```python
from build123d import *

# Parameters (mm, degrees)
SKETCH2_W               = 6.35
SKETCH2_H               = 50.8
SKETCH2_W_2             = 2.54
SKETCH2_W_3             = 31.75
SKETCH2_W_4             = 3.81
SKETCH2_W_5             = 12.7
BOSS_EXTRUDE2_DEPTH     = 73.66
CUT_EXTRUDE2_DEPTH      = 26.4
CUT_EXTRUDE2_DEPTH_BACK = 77.2
CUT_EXTRUDE3_DEPTH      = 22.86
CUT_EXTRUDE4_DEPTH      = 38.1


with BuildPart() as part:
    # Sketch2 → Boss-Extrude2 (new body)
    with BuildSketch(Plane.XY):
        with Locations((98.925952955, 12.684680338)):
            Rectangle(SKETCH2_W, SKETCH2_H)
        with Locations((105.275952955, 12.684680338)):
            Rectangle(SKETCH2_W, SKETCH2_H)
        with Locations((109.720952955, 12.684680338)):
            Rectangle(SKETCH2_W_2, SKETCH2_H)
        with Locations((79.875952955, 12.684680338)):
            Rectangle(SKETCH2_W_3, SKETCH2_H)
        with Locations((62.095952955, 12.684680338)):
            Rectangle(SKETCH2_W_4, SKETCH2_H)
        Polygon((-28.709047045, -38.115319662), (60.190952955, -38.115319662), (60.190952955, 63.484680338), (-28.709047045, 63.484680338), (-28.709047045, -12.715319662), align=None)
        with Locations((-31.884047045, 12.684680338)):
            Rectangle(SKETCH2_W, SKETCH2_H)
        with Locations((-50.934047045, 12.684680338)):
            Rectangle(SKETCH2_W_3, SKETCH2_H)
        with Locations((-69.984047045, 12.684680338)):
            Rectangle(SKETCH2_W, SKETCH2_H)
        with Locations((-76.334047045, 12.684680338)):
            Rectangle(SKETCH2_W, SKETCH2_H)
        with Locations((-85.859047045, 12.684680338)):
            Rectangle(SKETCH2_W_5, SKETCH2_H)
    extrude(amount=BOSS_EXTRUDE2_DEPTH)

    # Sketch4 → Cut-Extrude2 (cut, two sides)
    with BuildSketch(Plane(origin=(0, 38.084680338, 0), x_dir=(1, 0, 0), z_dir=(0, 1, 0))) as cut_extrude2_sk:
        with BuildLine():
            Line((-73.159047045, -60.96), (-73.159047045, -67.31))
            ThreePointArc((-73.159047045, -67.31), (-68.668918984, -65.450128061), (-66.809047045, -60.96))
            ThreePointArc((-66.809047045, -60.96), (-68.668918984, -56.469871939), (-73.159047045, -54.61))
            Line((-73.159047045, -54.61), (-73.159047045, -60.96))
        make_face()
        with BuildLine():
            Line((-79.50524406, -60.740265064), (-79.50524406, -61.179734936))
            ThreePointArc((-79.50524406, -61.179734936), (-77.57080311, -65.527155397), (-73.159047045, -67.31))
            Line((-73.159047045, -67.31), (-73.159047045, -60.96))
            Line((-73.159047045, -60.96), (-73.159047045, -54.61))
            ThreePointArc((-73.159047045, -54.61), (-77.57080311, -56.392844603), (-79.50524406, -60.740265064))
        make_face()
        with BuildLine():
            ThreePointArc((102.100952955, -54.61), (97.610824895, -56.469871939), (95.750952955, -60.96))
            ThreePointArc((95.750952955, -60.96), (97.610824895, -65.450128061), (102.100952955, -67.31))
            Line((102.100952955, -67.31), (102.100952955, -60.96))
            Line((102.100952955, -60.96), (102.100952955, -54.61))
        make_face()
        with BuildLine():
            ThreePointArc((108.450952955, -60.96), (106.591081016, -56.469871939), (102.100952955, -54.61))
            Line((102.100952955, -54.61), (102.100952955, -60.96))
            Line((102.100952955, -60.96), (102.100952955, -67.31))
            ThreePointArc((102.100952955, -67.31), (106.591081016, -65.450128061), (108.450952955, -60.96))
        make_face()
    extrude(amount=CUT_EXTRUDE2_DEPTH, mode=Mode.SUBTRACT)
    extrude(cut_extrude2_sk.sketch, amount=-CUT_EXTRUDE2_DEPTH_BACK, mode=Mode.SUBTRACT)

    # Sketch5 → Cut-Extrude3 (cut)
    with BuildSketch(Plane(origin=(0, 0, 0), x_dir=(-1, 0, 0), z_dir=(0, 0, -1))):
        Polygon((-60.190952955, -38.115319662), (-60.190952955, -12.715319662), (-110.990952955, -12.715319662), (-110.990952955, 38.084680338), (-60.190952955, 38.084680338), (-60.190952955, 63.484680338), (28.709047045, 63.484680338), (28.709047045, 38.084680338), (92.209047045, 38.084680338), (92.209047045, -12.715319662), (28.709047045, -12.715319662), (28.709047045, -38.115319662), align=None)
    extrude(amount=-CUT_EXTRUDE3_DEPTH, mode=Mode.SUBTRACT)

    # Sketch8 → Cut-Extrude4 (cut)
    with BuildSketch(Plane(origin=(0, 0, 22.86), x_dir=(-1, 0, 0), z_dir=(0, 0, -1))):
        Polygon((-104.640952955, -6.365319662), (-53.840952955, -6.365319662), (-53.840952955, -31.765319662), (22.359047045, -31.765319662), (22.359047045, -6.365319662), (85.859047045, -6.365319662), (85.859047045, 31.734680338), (22.359047045, 31.734680338), (22.359047045, 57.134680338), (-53.840952955, 57.134680338), (-53.840952955, 31.734680338), (-104.640952955, 31.734680338), align=None)
    extrude(amount=-CUT_EXTRUDE4_DEPTH, mode=Mode.SUBTRACT)


solid = part.part
```
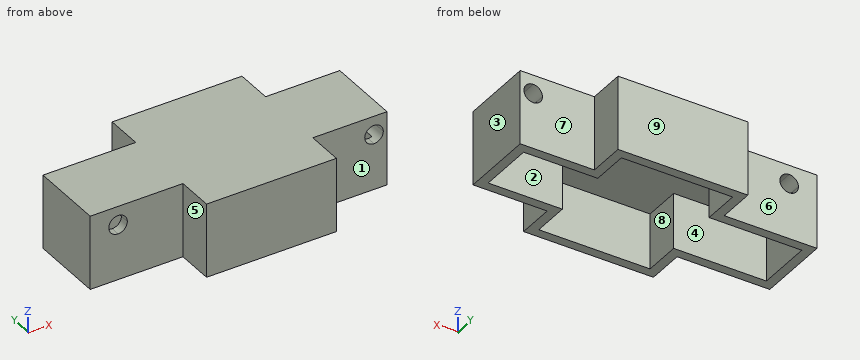
Could you check a few things on this model? Use its own coordinates, in mm. Face numbers are marked on the shaded views. A direction names the side the tool comes from. Give positions to 0.01 mm unless a question says otherwise; leave off trailing zeros. Write each loop counter-clockwise with the first axis right and the second up, starting at its lowest first coordinate (ties: lowest second). Pieces come first, ordered by that corner, then holes. Notation, with made-up numbers: (34.25, 6.5) - (93.25, 6.5) arc R9 ccw to (93.25, 10.5) - close; hole circle Ø5 at (-2.75, 39.25). An arc over 180 degrees is marked (long way). One line per item, written item: value. Start each with the question number.
Item 1: Imagine slicing it at C-C, the plane y = 4. List the corners of the cut face in (x, z) for me, and give its area (3 significant figures).
Item 2: Imagine slicing it at A-A, the plane z = 46.5. List the corners of the cut face in (x, y) for me.
Item 3: Imagine slicing it at B-B, the plane x = 81. List the corners of the cut face in (y, z) for me, and give its area (3 significant figures).
Item 4: Please list where these lines run through material, in increasing order: line 1 (Y direction, x = -10, z = 49); line 2 (X direction, y = 47, z = 48); line 3 (X direction, y = -9, z = 40). Write a range as from..to.
Item 5: If we mould it in two halves opening along X, with no side actions, what happens to the marked faces 1, 2, 3 and 4? For each: +X half, -X half, draft (parallel to the pull), parting line (faces both ways), or undercut.
Item 6: Which directions (+Z, -Z, +X, -X, +Y, -Y) give clear straight access to the entire face, cutting with the end or side of a thin tool? Please do the marked faces 5, 6, 7, 8 and 9.
Item 7: I'm going to push flat-ended pins straight in: pin 1 (8 mm diameter, centred on x = -35, z = 38, fed in from +Y); pin 2 (12.5 mm diameter, centred on y = -14, z = 41.5, fed in from -X); pin 3 (3 mm diameter, centred on x = -84, y = 14, fed in from -Z); pin 4 (7.5 mm diameter, centred on y = -27.5, z = 60, fed in from +X). Where does each tip first touch, or does it pass through?
Item 8: Imagine slicing it at D-D, the plane x = 44.5. List the corners of the cut face in (y, z) for me, and give its area (3 significant figures).
Geometry says:
1. outline: (-92.21, 22.86) - (-85.86, 22.86) - (-85.86, 60.96) - (-79.51, 60.96) - (-79.51, 61.18) arc R6.35 cw to (-66.81, 60.96) - (95.75, 60.96) arc R6.35 cw (long way) to (104.64, 55.14) - (104.64, 22.86) - (110.99, 22.86) - (110.99, 73.66) - (-92.21, 73.66) - close
1. area: 2,920 mm^2
2. outline: (-92.21, -12.72) - (-28.71, -12.72) - (-28.71, -38.12) - (60.19, -38.12) - (60.19, -12.72) - (110.99, -12.72) - (110.99, 38.08) - (60.19, 38.08) - (60.19, 63.48) - (-28.71, 63.48) - (-28.71, 38.08) - (-92.21, 38.08) - close; hole (-85.86, -6.37) - (-22.36, -6.37) - (-22.36, -31.77) - (53.84, -31.77) - (53.84, -6.37) - (104.64, -6.37) - (104.64, 31.73) - (53.84, 31.73) - (53.84, 57.13) - (-22.36, 57.13) - (-22.36, 31.73) - (-85.86, 31.73) - close
3. outline: (-12.72, 22.86) - (-6.37, 22.86) - (-6.37, 60.96) - (31.73, 60.96) - (31.73, 22.86) - (38.08, 22.86) - (38.08, 73.66) - (-12.72, 73.66) - close
3. area: 1,130 mm^2
4. line 1: -38.12..-31.77, 57.13..63.48
4. line 2: -28.71..-22.36, 53.84..60.19
4. line 3: -92.21..-22.36, 53.84..110.99
5. face 1: draft
5. face 2: undercut
5. face 3: +X half
5. face 4: undercut
6. face 5: +Z, -Z, -X, -Y
6. face 6: +Z, -Z, -X, +Y
6. face 7: +Z, -Z, +X, +Y
6. face 8: -Z
6. face 9: +Z, -Z, +X, -X, +Y
7. pin 1: y = 38.08
7. pin 2: x = -92.21
7. pin 3: z = 60.96
7. pin 4: x = 60.19
8. outline: (-38.12, 22.86) - (-31.77, 22.86) - (-31.77, 60.96) - (57.13, 60.96) - (57.13, 22.86) - (63.48, 22.86) - (63.48, 73.66) - (-38.12, 73.66) - close
8. area: 1,770 mm^2
